Can you work these out from the model? Positions are in its coordinate system, mm. Face numbers are marked on the shaded views. A direction names the side the tool comes from. Give positions to 0.01 mm unless a question says otherwise; leave off trailing zeros. Write each loop counter-clockwise with the first axis right and the second up, starting at its lowest first coordinate (ties: lowest second). Pieces come first, ordered by that corner, then holes. Notation, with made-up numbers: (16, 59.25) -> (63, 59.25) arc R24 cw to (63, 69.25) -> close; hole circle Ø9 at (57, 16). An arc over 180 degrees is marked (long way). One line per item, written item: value.
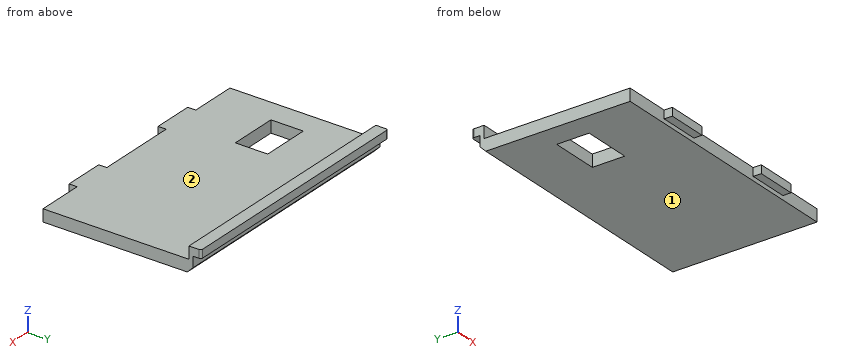
from build123d import *

# Parameters (mm, degrees)
SKETCH1_W           = 63
SKETCH1_H           = 37
BOSS_EXTRUDE1_DEPTH = 3
SKETCH2_W           = 10
SKETCH2_H           = 2
BOSS_EXTRUDE2_DEPTH = 2
SKETCH3_W           = 63
SKETCH3_H           = 1
BOSS_EXTRUDE3_DEPTH = 3
SKETCH4_W           = 12
SKETCH4_H           = 8
CUT_EXTRUDE1_DEPTH  = 4
SKETCH5_W           = 63
SKETCH5_H           = 2
BOSS_EXTRUDE4_DEPTH = 2
CHAMFER1_SIZE       = 1.4
FILLET1_R           = 0.5


with BuildPart() as part:
    # Sketch1 → Boss-Extrude1 (new body)
    with BuildSketch(Plane.XY):
        Rectangle(SKETCH1_W, SKETCH1_H)
    extrude(amount=BOSS_EXTRUDE1_DEPTH)

    # Sketch2 → Boss-Extrude2 (add)
    with BuildSketch(Plane.XZ.offset(18.5)):
        with Locations((-15, 2)):
            Rectangle(SKETCH2_W, SKETCH2_H)
        with Locations((15, 2)):
            Rectangle(SKETCH2_W, SKETCH2_H)
    extrude(amount=BOSS_EXTRUDE2_DEPTH)

    # Sketch3 → Boss-Extrude3 (add)
    with BuildSketch(Plane.XY.offset(3)):
        with Locations((0, 18)):
            Rectangle(SKETCH3_W, SKETCH3_H)
    extrude(amount=BOSS_EXTRUDE3_DEPTH)

    # Sketch4 → Cut-Extrude1 (cut, through all)
    with BuildSketch(Plane.XY.offset(3)):
        with Locations((-19.5, 0)):
            Rectangle(SKETCH4_W, SKETCH4_H)
    extrude(amount=-CUT_EXTRUDE1_DEPTH, mode=Mode.SUBTRACT)

    # Sketch5 → Boss-Extrude4 (add)
    with BuildSketch(Plane(origin=(0, 18.5, 0), x_dir=(1, 0, 0), z_dir=(0, 1, 0))):
        with Locations((0, -5)):
            Rectangle(SKETCH5_W, SKETCH5_H)
    extrude(amount=BOSS_EXTRUDE4_DEPTH)

    # Chamfer1
    chamfer1_edges = [part.edges().sort_by_distance(p)[0] for p in [
        (0, 18.5, 0),
    ]]
    chamfer(chamfer1_edges, length=CHAMFER1_SIZE)

    # Fillet1
    fillet1_edges = [part.edges().sort_by_distance(p)[0] for p in [
        (31.5, 20.5, 5),
        (-31.5, 20.5, 5),
    ]]
    fillet(fillet1_edges, radius=FILLET1_R)


solid = part.part
1) If we section it at A-A (x = -17.5): Write out the boundary of the cut face in (y, z), and give its area (3 significant figures).
Answer list:
outline: (-20.5, 1) -> (-18.5, 1) -> (-18.5, 0) -> (-4, 0) -> (-4, 3) -> (-20.5, 3) -> close; (4, 0) -> (17.1, 0) -> (18.5, 1.4) -> (18.5, 4) -> (20.5, 4) -> (20.5, 6) -> (17.5, 6) -> (17.5, 3) -> (4, 3) -> close
area: 97.0 mm^2
2) If we section it at B-B (z = 2.25): Write out the boundary of the cut face in (x, y), and give its area (4 significant figures).
Answer list:
outline: (-31.5, -18.5) -> (-20, -18.5) -> (-20, -20.5) -> (-10, -20.5) -> (-10, -18.5) -> (10, -18.5) -> (10, -20.5) -> (20, -20.5) -> (20, -18.5) -> (31.5, -18.5) -> (31.5, 18.5) -> (-31.5, 18.5) -> close; hole (-25.5, -4) -> (-13.5, -4) -> (-13.5, 4) -> (-25.5, 4) -> close
area: 2,275 mm^2
3) For the marked faces 1 and 2, which set-ups out of +Z, -Z, +X, -X, +Y, -Y let a thin tool reach every point of the face, with its end or its side?
Answer list:
face 1: -Z, +X, -X, +Y, -Y
face 2: +Z, +X, -X, -Y
4) Will these pins go through, and if not, where does the flat tip stop? pin 1 (1.3 mm diameter, centred on x = 1.5, z = 3, fed in from +Y); pin 2 (0.6 mm diameter, centred on y = -19.5, z = 2.5, fed in from -X); pin 3 (1.6 mm diameter, centred on x = -2, y = 19.5, fed in from -Z).
Answer list:
pin 1: stops at y = 18.5
pin 2: stops at x = -20
pin 3: stops at z = 4
5) If we section it at D-D (x = 2.5): Write out the boundary of the cut face in (y, z).
Answer list:
outline: (-18.5, 0) -> (17.1, 0) -> (18.5, 1.4) -> (18.5, 4) -> (20.5, 4) -> (20.5, 6) -> (17.5, 6) -> (17.5, 3) -> (-18.5, 3) -> close
6) If we section it at C-C (y = 2): Write out the boundary of the cut face in (x, z).
Answer list:
outline: (-31.5, 0) -> (-25.5, 0) -> (-25.5, 3) -> (-31.5, 3) -> close; (-13.5, 0) -> (31.5, 0) -> (31.5, 3) -> (-13.5, 3) -> close
7) I need wall thicknesses on L1, parallel to Z at x = -1.5, y = -1; L2, parallel to Y at x = 10, z = 5.5; L3, parallel to Y at x = 23, z = 3.5. Which ranges of each line are inside material? Lowest first, please.
Answer list:
L1: z = 0 to 3
L2: y = 17.5 to 20.5
L3: y = 17.5 to 18.5
